The listing builds one solid part. Answer for the finished solid, in the listing's coordinates (mm). Coordinates: 2 decimals unless noted, no trailing zeros. Order: outer loops, then holes, each group sorted by start corner. A loop starts at its lowest first (then second) coordinate and runs counter-clockwise, first axis right, second up. Notation, with made-up numbers: (72, 74) -> (107, 74) arc R19 ccw to (107, 104) -> close; hole circle Ø11 at (58, 78). An arc over 180 degrees is marked (long way). Answer in a Markdown table with one row per item.
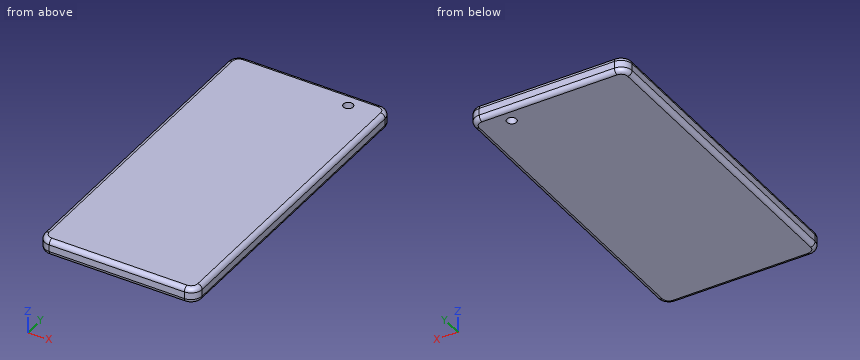
Autodesk Inventor part; units mm, degrees
ref_plane "YZ Plane" through (0, 0, 0) normal (1, 0, 0) x (0, 1, 0)
ref_plane "XZ Plane" through (0, 0, 0) normal (0, 1, 0) x (-1, 0, 0)
ref_plane "XY Plane" through (0, 0, 0) normal (0, 0, 1) x (1, 0, 0)
ref_plane "Work Plane1" through (0, 0, 24.8) normal (0, 0, 1) x (1, 0, 0)
sketch "Sketch1" plane through (0, 0, 24.8) normal (0, 0, 1) x (1, 0, 0)
  circle A0 centre (0, 0) radius 2.1512
  line L0 (10.2, 7.3) -> (-50.7, 7.3)
  line L1 (-55.7, 2.3) -> (-55.7, -132.8)
  line L2 (-50.7, -137.8) -> (10.2, -137.8)
  line L3 (15.2, -132.8) -> (15.2, 2.3)
  arc A1 (-50.7, 7.3) -> (-55.7, 2.3) centre (-50.7, 2.3) ccw
  arc A2 (10.2, -137.8) -> (15.2, -132.8) centre (10.2, -132.8) ccw
  arc A3 (-55.7, -132.8) -> (-50.7, -137.8) centre (-50.7, -132.8) ccw
  arc A4 (15.2, 2.3) -> (10.2, 7.3) centre (10.2, 2.3) ccw
  point P0 (-55.7, -137.8)
  point P1 (-55.7, 7.3)
  point P2 (15.2, -137.8)
  dimension "d0" = 70.9
  dimension "d1" = 145.1
  dimension "d2" = 15.2
  dimension "d3" = 7.3
  dimension "d5" = 5
extrude "Extrusion1" add sketch "Sketch1" along normal blind 7.1
fillet "Fillet1" radius 2 16 edges at (13.7355, 5.8355, 31.9) (-20.25, 7.3, 31.9) (-54.2355, 5.8355, 31.9) (-55.7, -65.25, 31.9) (-54.2355, -136.3355, 31.9) (-20.25, -137.8, 31.9) (13.7355, -136.3355, 31.9) (15.2, -65.25, 31.9) (-54.2355, 5.8355, 24.8) (-55.7, -65.25, 24.8) (-54.2355, -136.3355, 24.8) (-20.25, -137.8, 24.8) (13.7355, -136.3355, 24.8) (15.2, -65.25, 24.8) (13.7355, 5.8355, 24.8) (-20.25, 7.3, 24.8)
properties part number "100_Huawei_P9"
(1) A cutting plane is placed at A-A, the plane y = 0. Determine the outline of the cut face in (x, z), then the cut area to 3 significant figures.
Check values:
| item | result |
|---|---|
| outline | (-55.7, 26.8) arc R2 ccw to (-53.7, 24.8) -> (-2.15, 24.8) -> (-2.15, 31.9) -> (-53.7, 31.9) arc R2 ccw to (-55.7, 29.9) -> close; (2.15, 24.8) -> (13.2, 24.8) arc R2 ccw to (15.2, 26.8) -> (15.2, 29.9) arc R2 ccw to (13.2, 31.9) -> (2.15, 31.9) -> close |
| area | 469 mm² |
(2) Find the intervals of material crossed by line 1 along Y through (x, z) = (0, 27.5); line 2 along X through (y, z) = (-34, 30); line 3 along Y through (x, z) = (1, 27.5), in increasing order. Write a range as from..to.
Check values:
| item | result |
|---|---|
| line 1 | -137.8..-2.15, 2.15..7.3 |
| line 2 | -55.7..15.2 |
| line 3 | -137.8..-1.9, 1.9..7.3 |
(3) A flat-ended cylindrical pin translates along its axis: pin 1 (2 mm diameter, centred on y = -57, z = 25.5, fed in from +X). Find the tip coordinate at first contact, or state that the pin passes through.
Check values:
| item | result |
|---|---|
| pin 1 | x = 15.18 |
(4) A cutting plane is placed at B-B, the plane x = 0. Determine the outline of the cut face in (y, z), then the cut area to 3 significant figures.
Check values:
| item | result |
|---|---|
| outline | (-137.8, 26.8) arc R2 ccw to (-135.8, 24.8) -> (-2.15, 24.8) -> (-2.15, 31.9) -> (-135.8, 31.9) arc R2 ccw to (-137.8, 29.9) -> close; (2.15, 24.8) -> (5.3, 24.8) arc R2 ccw to (7.3, 26.8) -> (7.3, 29.9) arc R2 ccw to (5.3, 31.9) -> (2.15, 31.9) -> close |
| area | 996 mm² |
